The model under review builds one solid part; all positions refer to its coordinate system, in mm. Face numbers are marked on the shaded views. A direction names the side the tool comes from. Coordinates: 2 decimals unless noted, no trailing zeros. Write each loop counter-clockwise with the first axis right and the second up, starting at its lowest first coordinate (ties: lowest second). Pieces come first, ordered by that corner, then holes.
```python
from build123d import *

# Parameters (mm, degrees)
PAD_DEPTH     = 20.07
POCKET_DEPTH  = 18.42
SKETCH002_R   = 3
HOLE_DEPTH    = 25
SKETCH003_R   = 3
HOLE001_DEPTH = 25
SKETCH004_R   = 3
HOLE002_DEPTH = 25
SKETCH005_R   = 3
HOLE003_DEPTH = 25
SKETCH006_R   = 3
HOLE004_DEPTH = 25
SKETCH007_R   = 3
HOLE005_DEPTH = 25
SKETCH008_R   = 3
HOLE006_DEPTH = 25
FILLET_R      = 1.5
SKETCH009_R   = 3
HOLE007_DEPTH = 25
SKETCH010_R   = 3
HOLE008_DEPTH = 25
SKETCH011_R   = 3
HOLE009_DEPTH = 25
SKETCH012_R   = 3
HOLE010_DEPTH = 25
SKETCH013_R   = 3
HOLE011_DEPTH = 25
SKETCH014_R   = 3
HOLE012_DEPTH = 25
SKETCH015_R   = 3
HOLE013_DEPTH = 25


with BuildPart() as part:
    # Sketch → Pad (new body)
    with BuildSketch(Plane.XY):
        with BuildLine():
            Line((26.468666, 48.305671), (88.278666, 48.305671))
            ThreePointArc((97.278666, 39.305671), (94.642627, 45.669632), (88.278666, 48.305671))
            Line((97.278666, 39.305671), (97.278666, 19.715671))
            ThreePointArc((88.278666, 10.715671), (94.642627, 13.351709), (97.278666, 19.715671))
            Line((88.278666, 10.715671), (26.468666, 10.715671))
            ThreePointArc((17.468666, 19.715671), (20.104705, 13.351709), (26.468666, 10.715671))
            Line((17.468666, 19.715671), (17.468666, 39.305671))
            ThreePointArc((26.468666, 48.305671), (20.104705, 45.669632), (17.468666, 39.305671))
        make_face()
    extrude(amount=PAD_DEPTH)

    # Sketch001 (on Face9 of Pad) → Pocket (cut)
    with BuildSketch(Plane(origin=(0, 0, 0), x_dir=(1, 0, 0), z_dir=(0, 0, -1))):
        with BuildLine():
            Line((26.978666, -11.220671), (87.768666, -11.220671))
            ThreePointArc((96.768666, -20.220671), (94.132627, -13.856709), (87.768666, -11.220671))
            Line((96.768666, -20.220671), (96.768666, -38.800671))
            ThreePointArc((87.768666, -47.800671), (94.132627, -45.164632), (96.768666, -38.800671))
            Line((87.768666, -47.800671), (26.978666, -47.800671))
            ThreePointArc((17.978666, -38.800671), (20.614705, -45.164632), (26.978666, -47.800671))
            Line((17.978666, -38.800671), (17.978666, -20.220671))
            ThreePointArc((26.978666, -11.220671), (20.614705, -13.856709), (17.978666, -20.220671))
        make_face()
    extrude(amount=-POCKET_DEPTH, mode=Mode.SUBTRACT)

    # Sketch002 (on Face5 of Pocket) → Hole (cut)
    with BuildSketch(Plane.XY.offset(20.07)):
        with Locations((57.373666, 38.908171)):
            Circle(SKETCH002_R)
    extrude(amount=-HOLE_DEPTH, mode=Mode.SUBTRACT)

    # Sketch003 (on Face5 of Hole) → Hole001 (cut)
    with BuildSketch(Plane.XY.offset(20.07)):
        with Locations((47.135866, 38.908171)):
            Circle(SKETCH003_R)
    extrude(amount=-HOLE001_DEPTH, mode=Mode.SUBTRACT)

    # Sketch004 (on Face5 of Hole001) → Hole002 (cut)
    with BuildSketch(Plane.XY.offset(20.07)):
        with Locations((36.925066, 38.908171)):
            Circle(SKETCH004_R)
    extrude(amount=-HOLE002_DEPTH, mode=Mode.SUBTRACT)

    # Sketch005 (on Face5 of Hole002) → Hole003 (cut)
    with BuildSketch(Plane.XY.offset(20.07)):
        with Locations((26.714266, 38.908171)):
            Circle(SKETCH005_R)
    extrude(amount=-HOLE003_DEPTH, mode=Mode.SUBTRACT)

    # Sketch006 (on Face5 of Hole003) → Hole004 (cut)
    with BuildSketch(Plane.XY.offset(20.07)):
        with Locations((67.557466, 38.908171)):
            Circle(SKETCH006_R)
    extrude(amount=-HOLE004_DEPTH, mode=Mode.SUBTRACT)

    # Sketch007 (on Face5 of Hole004) → Hole005 (cut)
    with BuildSketch(Plane.XY.offset(20.07)):
        with Locations((77.768266, 38.908171)):
            Circle(SKETCH007_R)
    extrude(amount=-HOLE005_DEPTH, mode=Mode.SUBTRACT)

    # Sketch008 (on Face5 of Hole005) → Hole006 (cut)
    with BuildSketch(Plane.XY.offset(20.07)):
        with Locations((87.979066, 38.908171)):
            Circle(SKETCH008_R)
    extrude(amount=-HOLE006_DEPTH, mode=Mode.SUBTRACT)

    # Fillet
    fillet_edges = [part.edges().sort_by_distance(p)[0] for p in [
        (57.373666, 48.305671, 20.07),
    ]]
    fillet(fillet_edges, radius=FILLET_R)

    # Sketch009 (on Face8 of Fillet) → Hole007 (cut)
    with BuildSketch(Plane.XY.offset(20.07)):
        with Locations((57.373666, 20.113171)):
            Circle(SKETCH009_R)
    extrude(amount=-HOLE007_DEPTH, mode=Mode.SUBTRACT)

    # Sketch010 (on Face8 of Hole007) → Hole008 (cut)
    with BuildSketch(Plane.XY.offset(20.07)):
        with Locations((47.135866, 20.113171)):
            Circle(SKETCH010_R)
    extrude(amount=-HOLE008_DEPTH, mode=Mode.SUBTRACT)

    # Sketch011 (on Face8 of Hole008) → Hole009 (cut)
    with BuildSketch(Plane.XY.offset(20.07)):
        with Locations((36.925066, 20.113171)):
            Circle(SKETCH011_R)
    extrude(amount=-HOLE009_DEPTH, mode=Mode.SUBTRACT)

    # Sketch012 (on Face8 of Hole009) → Hole010 (cut)
    with BuildSketch(Plane.XY.offset(20.07)):
        with Locations((26.714266, 20.113171)):
            Circle(SKETCH012_R)
    extrude(amount=-HOLE010_DEPTH, mode=Mode.SUBTRACT)

    # Sketch013 (on Face8 of Hole010) → Hole011 (cut)
    with BuildSketch(Plane.XY.offset(20.07)):
        with Locations((67.557466, 20.113171)):
            Circle(SKETCH013_R)
    extrude(amount=-HOLE011_DEPTH, mode=Mode.SUBTRACT)

    # Sketch014 (on Face8 of Hole011) → Hole012 (cut)
    with BuildSketch(Plane.XY.offset(20.07)):
        with Locations((77.768266, 20.113171)):
            Circle(SKETCH014_R)
    extrude(amount=-HOLE012_DEPTH, mode=Mode.SUBTRACT)

    # Sketch015 (on Face8 of Hole012) → Hole013 (cut)
    with BuildSketch(Plane.XY.offset(20.07)):
        with Locations((87.979066, 20.113171)):
            Circle(SKETCH015_R)
    extrude(amount=-HOLE013_DEPTH, mode=Mode.SUBTRACT)


solid = part.part
```
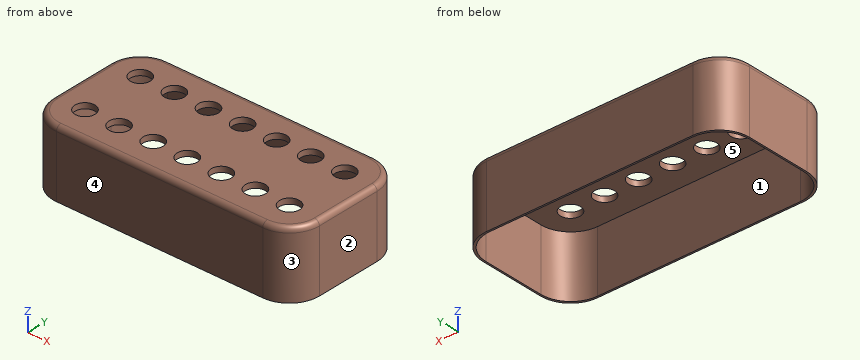
Item 1: Mouldability with a two-part tool opening along X and no side actions: class the marked faces 3, 4 and 5 as pulls with the +X half, pulls with the -X half, needs draft (parallel to the pull), parting line crosses it, or undercut.
Solved:
face 3: pulls with the +X half
face 4: needs draft
face 5: undercut
Item 2: To check wall thickness, follow line 1 along X through (y, z) = (28.5, 16.5); line 2 along Y through (x, z) = (78.5, 12); line 3 along Z through (x, y) = (49, 26.5). State the ranges of each line that lie inside material, in increasing order.
Solved:
line 1: x = 17.47 to 17.98, 96.77 to 97.28
line 2: y = 10.72 to 11.22, 47.8 to 48.31
line 3: z = 18.42 to 20.07
Item 3: Machinability: for the marked faces 1 and 2, which of the approach directions +Z, -Z, +X, -X, +Y, -Y give a long, thin tool a straight path to every point of the face, cutting with its end or side? Answer none if there is none.
Solved:
face 1: -Z
face 2: +Z, -Z, +X, +Y, -Y
Item 4: For pin 1 (5 mm diameter, centred on x = 77.77, y = 38.91, fed in from +Z); pin 2 (18.5 mm diameter, centred on x = 39, y = 29, fed in from -Z); pin 3 (8 mm diameter, centred on x = 87.98, y = 20.11, fed in from +Z), all flat-tipped, find the tip position at first contact; note any pin that passes through.
Solved:
pin 1: passes through
pin 2: stops at z = 18.42
pin 3: stops at z = 20.07
Item 5: Take a section at D-D, the plane x = 45. Write out the cut boundary in (y, z).
Solved:
outline: (10.72, 0) - (11.22, 0) - (11.22, 18.42) - (18.01, 18.42) - (18.01, 20.07) - (12.22, 20.07) arc R1.5 ccw to (10.72, 18.57) - close; (22.22, 18.42) - (36.8, 18.42) - (36.8, 20.07) - (22.22, 20.07) - close; (41.01, 18.42) - (47.8, 18.42) - (47.8, 0) - (48.31, 0) - (48.31, 18.57) arc R1.5 ccw to (46.81, 20.07) - (41.01, 20.07) - close
Item 6: Take a section at C-C, the plane z = 16.5. Write out the cut boundary in (x, y).
Solved:
outline: (17.47, 19.72) arc R9 ccw to (26.47, 10.72) - (88.28, 10.72) arc R9 ccw to (97.28, 19.72) - (97.28, 39.31) arc R9 ccw to (88.28, 48.31) - (26.47, 48.31) arc R9 ccw to (17.47, 39.31) - close; hole (17.98, 20.22) arc R9 ccw to (26.98, 11.22) - (87.77, 11.22) arc R9 ccw to (96.77, 20.22) - (96.77, 38.8) arc R9 ccw to (87.77, 47.8) - (26.98, 47.8) arc R9 ccw to (17.98, 38.8) - close
Item 7: Take a section at B-B, the plane x = 73. Write out the cut boundary in (y, z), plus the area to 3 significant figures.
Solved:
outline: (10.72, 0) - (11.22, 0) - (11.22, 18.42) - (47.8, 18.42) - (47.8, 0) - (48.31, 0) - (48.31, 18.57) arc R1.5 ccw to (46.81, 20.07) - (12.22, 20.07) arc R1.5 ccw to (10.72, 18.57) - close
area: 79.7 mm2
Item 8: Take a section at A-A, the plane y = 30. Write out the cut boundary in (x, z).
Solved:
outline: (17.47, 0) - (17.98, 0) - (17.98, 18.42) - (96.77, 18.42) - (96.77, 0) - (97.28, 0) - (97.28, 18.57) arc R1.5 ccw to (95.78, 20.07) - (18.97, 20.07) arc R1.5 ccw to (17.47, 18.57) - close
